```python
from build123d import *

# Parameters (mm, degrees)
SKETCH1_R           = 3.1115
BOSS_EXTRUDE1_DEPTH = 20.32
SKETCH2_R           = 1.905
BOSS_EXTRUDE2_DEPTH = 1.27
SKETCH3_R           = 4.27
CUT_EXTRUDE1_DEPTH  = 10.16


with BuildPart() as part:
    # Sketch1 → Boss-Extrude1 (new body)
    with BuildSketch(Plane.XY):
        with BuildLine():
            Line((-9.694539288, -3.646539288), (-12.7, -3.646539288))
            Line((-12.7, -3.646539288), (-12.7, -4.916539288))
            Line((-12.7, -4.916539288), (12.7, -4.916539288))
            Line((12.7, -4.916539288), (12.7, -3.646539288))
            Line((12.7, -3.646539288), (9.694539288, -3.646539288))
            ThreePointArc((9.694539288, -3.646539288), (7.11604663, -2.578492658), (6.048, 0))
            ThreePointArc((6.048, 0), (0, 6.048), (-6.048, 0))
            ThreePointArc((-6.048, 0), (-7.11604663, -2.578492658), (-9.694539288, -3.646539288))
        make_face()
        Circle(SKETCH1_R, mode=Mode.SUBTRACT)
    extrude(amount=BOSS_EXTRUDE1_DEPTH)

    # Sketch2 → Boss-Extrude2 (add)
    with BuildSketch(Plane(origin=(0, 0, 0), x_dir=(-1, 0, 0), z_dir=(0, 0, -1))):
        with BuildLine():
            Line((12.7, -4.916539288), (12.7, -3.646539288))
            Line((12.7, -3.646539288), (9.694539288, -3.646539288))
            ThreePointArc((9.694539288, -3.646539288), (7.11604663, -2.578492658), (6.048, 0))
            ThreePointArc((6.048, 0), (0, 6.048), (-6.048, 0))
            ThreePointArc((-6.048, 0), (-7.11604663, -2.578492658), (-9.694539288, -3.646539288))
            Line((-9.694539288, -3.646539288), (-12.7, -3.646539288))
            Line((-12.7, -3.646539288), (-12.7, -4.916539288))
            Line((-12.7, -4.916539288), (12.7, -4.916539288))
        make_face()
        Circle(SKETCH2_R, mode=Mode.SUBTRACT)
    extrude(amount=BOSS_EXTRUDE2_DEPTH)

    # Sketch3 → Cut-Extrude1 (cut)
    with BuildSketch(Plane.XY.offset(20.32)):
        Circle(SKETCH3_R)
    extrude(amount=-CUT_EXTRUDE1_DEPTH, mode=Mode.SUBTRACT)


solid = part.part
```
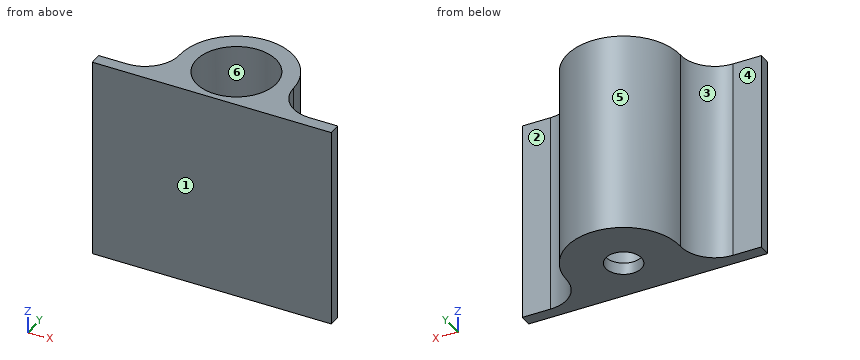
Work out the finished part from the listing and answer in its coordinate system (mm). Face numbers are marked on the shaded views. A direction names the side the tool comes from. Round coordinates to 2 decimals unless told otherwise and drop trailing zeros. Loops run counter-clockwise (first coordinate to the right, second up) from the corner with the lowest first, then second, coordinate; pieces in that order, holes last.
(1) For the marked faces 1 and 2, determine the directions among +Z, -Z, +X, -X, +Y, -Y from which every point of the face is accessible in a straight line to the end or side of a thin tool.
Computed values:
face 1: +Z, -Z, +X, -X, -Y
face 2: +Z, -Z, +X, +Y
(2) The part is cut by section D-D, the plane z = 1. Give the vertices of the cut face in (x, y).
Computed values:
outline: (-12.7, -4.92) - (12.7, -4.92) - (12.7, -3.65) - (9.69, -3.65) arc R3.65 cw to (6.05, 0) arc R6.05 ccw to (-6.05, 0) arc R3.65 cw to (-9.69, -3.65) - (-12.7, -3.65) - close; hole circle Ø6.22 at (0, 0)
(3) Find the intervals of material crossed by L1, parallel to Y at x = 0, z = 14.5; L2, parallel to Y at x = 0, z = 6.75; L3, parallel to X at y = 0, z = 4.75, in increasing order.
Computed values:
L1: y = -4.92 to -4.27, 4.27 to 6.05
L2: y = -4.92 to -3.11, 3.11 to 6.05
L3: x = -6.05 to -3.11, 3.11 to 6.05
(4) The part is cut by section B-B, the plane x = 0. Give the vertices of the cut face in (y, z) (1 decimal), and give its area (3 significant figures).
Computed values:
outline: (-4.9, -1.3) - (-1.9, -1.3) - (-1.9, 0) - (-3.1, 0) - (-3.1, 10.2) - (-4.3, 10.2) - (-4.3, 20.3) - (-4.9, 20.3) - close; (1.9, -1.3) - (6, -1.3) - (6, 20.3) - (4.3, 20.3) - (4.3, 10.2) - (3.1, 10.2) - (3.1, 0) - (1.9, 0) - close
area: 81.9 mm2
(5) The part is cut by section A-A, the plane z = 11.75. Give the vertices of the cut face in (x, y).
Computed values:
outline: (-12.7, -4.92) - (12.7, -4.92) - (12.7, -3.65) - (9.69, -3.65) arc R3.65 cw to (6.05, 0) arc R6.05 ccw to (-6.05, 0) arc R3.65 cw to (-9.69, -3.65) - (-12.7, -3.65) - close; hole circle Ø8.54 at (0, 0)
(6) The mould has two halves that part along X. Classify the marked faces 3, 4, 5 and 6: pulls with the +X half, pulls with the -X half, needs draft (parallel to the pull), parting line crosses it, or undercut.
Computed values:
face 3: pulls with the -X half
face 4: needs draft
face 5: parting line crosses it
face 6: undercut
(7) Each of these flat-tipped pins is pushed along its axis until it touches: P1, Ø3.5, axis at x = -10.5, z = 14.5, coming from the +Y side; P2, Ø6, axis at y = 4.5, z = 7, coming from the -X side; P3, Ø3, axis at x = -0.5, y = -0.5, coming from the +Z side. Where does it stop, or does it pass through?
Computed values:
P1: stops at y = -3.52
P2: stops at x = -5.86
P3: stops at z = 0
(8) The part is cut by section C-C, the plane y = -0.5. Give the vertices of the cut face in (x, z), and give its area (3 significant figures).
Computed values:
outline: (-6.08, -1.27) - (-1.84, -1.27) - (-1.84, 0) - (-3.07, 0) - (-3.07, 10.16) - (-4.24, 10.16) - (-4.24, 20.32) - (-6.08, 20.32) - close; (1.84, -1.27) - (6.08, -1.27) - (6.08, 20.32) - (4.24, 20.32) - (4.24, 10.16) - (3.07, 10.16) - (3.07, 0) - (1.84, 0) - close
area: 109 mm2
